Autodesk Inventor part; units mm, degrees
ref_plane "YZ Plane" through (0, 0, 0) normal (1, 0, 0) x (0, 1, 0)
ref_plane "XZ Plane" through (0, 0, 0) normal (0, 1, 0) x (-1, 0, 0)
ref_plane "XY Plane" through (0, 0, 0) normal (0, 0, 1) x (1, 0, 0)
sketch "Эскиз1" plane through (0, 0, 0) normal (0, 0, 1) x (1, 0, 0)
  line L0 (0, 0) -> (20, 0)
  line L1 (20, 0) -> (20, 30)
  line L2 (20, 30) -> (0, 30)
  line L3 (0, 30) -> (0, 0)
  dimension "d0" = 20
  dimension "d1" = 30
revolve "Вращение1" add sketch "Эскиз1" angle 360 about axis through (0, 0, 0) along (1, 0, 0)
sketch "Эскиз3" plane through (0, 0, 0) normal (0, 0, 1) x (1, 0, 0)
  line L0 (0, -30) -> (0, 30) construction
  line L1 (0, 26.5) -> (5, 26.5)
  line L2 (5, 26.5) -> (5, 21.5)
  line L3 (5, 21.5) -> (0, 21.5)
  line L4 (0, 21.5) -> (0, 26.5)
  line L5 (0, 18.5) -> (5, 18.5)
  line L6 (5, 18.5) -> (5, 13.5)
  line L7 (5, 13.5) -> (0, 13.5)
  line L8 (0, 13.5) -> (0, 18.5)
  line L9 (0, 0) -> (20, 0)
  line L10 (20, -30) -> (20, 30)
  dimension "d9" = 5
  dimension "d10" = 5
  dimension "d11" = 3
  dimension "d12" = 13.5
revolve "Вращение2" cut sketch "Эскиз3" angle 360 about axis through (0, 0, 0) along (1, 0, 0)
properties part number "711115"
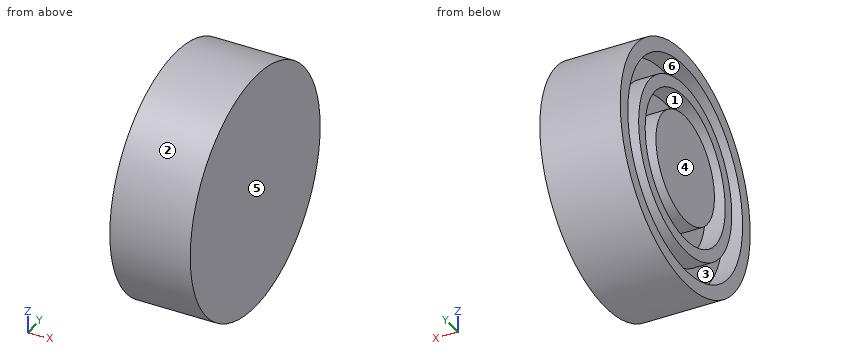
Build history of the part. All positions in model axes, mm. Face numbers are marked on the shaded views. A direction names the side the tool comes from. Give positions to 0.01 mm unless a question says otherwise; leave off trailing zeros. Write each loop counter-clockwise with the first axis right and the second up, starting at its lowest first coordinate (ties: lowest second). Pieces come first, ordered by that corner, then holes. Notation, with made-up numbers: (83.25, 62.25) - (114.25, 62.25) arc R31 cw to (114.25, 95.25) - close; hole circle Ø2 at (41.25, -4.5). An arc over 180 degrees is marked (long way). Use one line per item in the form item = value. Start each with the question number.
1. Band-saw the part on B-B on y = 0. Write the cut outline in (x, z), plus the area to 3 significant figures.
2. Band-saw the part on A-A on x = 2. Write the cut outline in (y, z).
3. Band-saw the part on D-D on x = 11.5. Write the cut outline in (y, z).
4. Two-plate mould, pull along Z, no slides. Class the marked faces 1, 2, 3 and 4: released by +Z, released by -Z, zero draft, split by the parting line, or undercut.
5. Probe line 1 (Z direction, x = 1.75, y = 0); line 2 (X direction, y = 22, z = -12.5); line 3 (Y direction, x = 17.5, z = 1). List the from-to ranges inside material, lowest first. Write a range as [from, to].
6. 3-axis set-ups, long thin cutter, end or side, ignore diameter. For the marked faces 5 and 6: which of +Z, -Z, +X, -X, +Y, -Y reach the whole face in a straight line?
7. Drop flat-ended pins along their axis: pin 1 Ø12 at (y, z) = (2, 23) entering from -X; pin 2 Ø10 at (x, z) = (2.5, 20) entering from +Y; pin 3 Ø12 at (x, y) = (6.5, 4.5) entering from +Z; pin 4 Ø1 at (x, z) = (16, -18.5) entering from -Y. Give the stop position or say it passes through.
Conclusion:
q1.outline = (0, -30) - (20, -30) - (20, 30) - (0, 30) - (0, 26.5) - (5, 26.5) - (5, 21.5) - (0, 21.5) - (0, 18.5) - (5, 18.5) - (5, 13.5) - (0, 13.5) - (0, -13.5) - (5, -13.5) - (5, -18.5) - (0, -18.5) - (0, -21.5) - (5, -21.5) - (5, -26.5) - (0, -26.5) - close
q1.area = 1,100 mm²
q2.outline = circle Ø60 at (0, 0); circle Ø43 at (0, 0); circle Ø27 at (0, 0); hole circle Ø53 at (0, 0); hole circle Ø37 at (0, 0)
q3.outline = circle Ø60 at (0, 0)
q4.face_1 = undercut
q4.face_2 = split by the parting line
q4.face_3 = undercut
q4.face_4 = zero draft
q5.line_1 = [-30, -26.5], [-21.5, -18.5], [-13.5, 13.5], [18.5, 21.5], [26.5, 30]
q5.line_2 = [5, 20]
q5.line_3 = [-29.98, 29.98]
q6.face_5 = +Z, -Z, +X, +Y, -Y
q6.face_6 = -X
q7.pin_1 = 0
q7.pin_2 = 25.98
q7.pin_3 = 30
q7.pin_4 = -24
